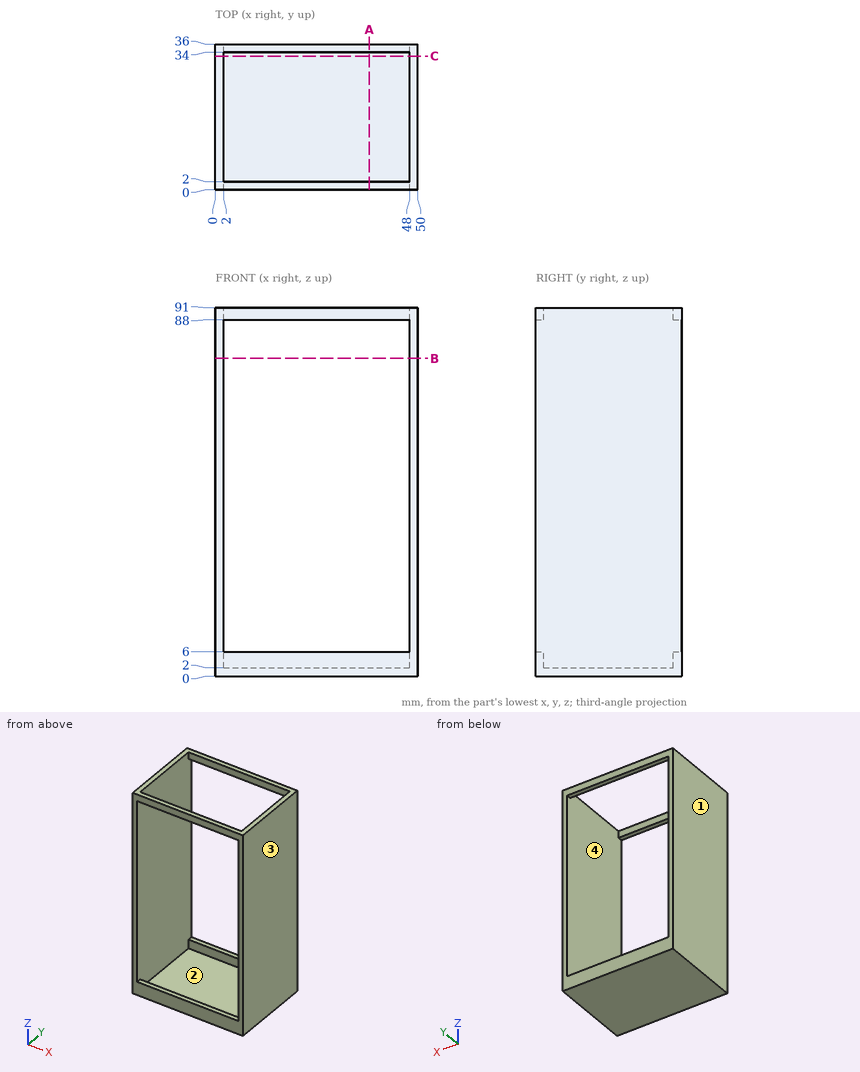
Here's the drawing with two shaded views (mm, measured from the low corner). I have some questions. Give positions to 0.01 mm unless a question says otherwise; leave off trailing zeros. Loops run counter-clockwise (first coordinate to the right, second up) from the corner with the lowest first, then second, coordinate; pieces in that order, holes last. Notation, with made-up numbers: M 81.25,60 L 86.25,60 A23 cw 86.25,90 Z; hole C 33.25,-17.75 d3. An arc over 180 degrees is marked long. Use one line per item in the form item = value. Start each with the question number.
(1) Thinking about a two-plate mould opening in X: for the marked faces 1, 2, 3 and 4, which applies, released by +X, released by -X, zero draft, split by the parting line, or undercut?
(2) I want a section at A-A, the plane x = 38. Write out the boundary of the cut face in (y, z), and give its area (3 significant figures).
(3) I want a section at B-B, the plane z = 78.5. Write out the boundary of the cut face in (x, y).
(4) Please list where these lines run through material, in increasing order: line 1 (X direction, y = 21.5, z = 59); line 2 (Y direction, x = 19.5, z = 4); line 3 (Z direction, x = 38, y = 30).
(5) I want a section at C-C, the plane y = 33. Write out the boundary of the cut face in (x, z), and give its area (3 significant figures).
(6) I'm going to push a flat-ended pin straight in: P1, Ø16, axis at x = 20, y = 14.5, coming from the +Z side. Where does the tip first touch, or does it pass through?
Worked out:
q1.face_1 = released by -X
q1.face_2 = undercut
q1.face_3 = released by +X
q1.face_4 = undercut
q2.outline = M 0,0 L 36,0 L 36,6 L 34,6 L 34,2 L 2,2 L 2,6 L 0,6 Z; M 0,88 L 2,88 L 2,91 L 0,91 Z; M 34,88 L 36,88 L 36,91 L 34,91 Z
q2.area = 100 mm²
q3.outline = M 0,0 L 2,0 L 2,36 L 0,36 Z; M 48,0 L 50,0 L 50,36 L 48,36 Z
q4.line_1 = 0 to 2, 48 to 50
q4.line_2 = 0 to 2, 34 to 36
q4.line_3 = 0 to 2
q5.outline = M 0,0 L 50,0 L 50,91 L 48,91 L 48,2 L 2,2 L 2,91 L 0,91 Z
q5.area = 456 mm²
q6.P1 = 2
